Check sheet for the modelled part. Datum: model origin and axes. Units: mm. A direction names the side the tool comes from. Round coordinates to 2 decimals unless told otherwise and drop trailing zeros. Loops run counter-clockwise (first coordinate to the right, second up) from the corner with the lowest first, then second, coordinate; pieces in that order, holes last. Notation, with made-up numbers: M 35.25,14 L 93.25,14 A27 cw 93.25,53 Z; hole C -2,51.25 d6. An arc over 180 degrees is marked long. Write item = value, one per line. Start each with the question number.
(1) Cross-section at A-A on x = 17.5. Record the boundary of the cut face in (y, z), plus the area to 3 significant figures.
(2) Mould release check, pull along Y, two halves, no side actions. Record for faces 1 (the face through (-33.65, -293.89, 14.79)), 2 (the face through (16, -148, 30)), 3 (the face through (35.88, -159.72, 14.79)): pulls with the +Y half, pulls with the -Y half, needs draft (parallel to the pull), parting line crosses it, or undercut.
(3) Cross-section at C-C on x = 0. Record the boundary of the cut face in (y, z), plus the area to 3 significant figures.
(4) Set-up check for faces 4 (the face through (18, -162, 0)), 5 (the face through (13.163, -144.473, 14.79)): record each of +Z, -Z, +X, -X, +Y, -Y from which the full face is reachable in a straight line by a thin tool's end or side.
(5) Cross-section at B-B on z = 21.25. Record the boundary of the cut face in (x, y), plus the area to 3 significant figures.
(6) Cross-section at D-D on y = 0. Record the boundary of the cut face in (x, z).
(7) Scan lines: L1, parallel to X at y = -142, z = 20; L2, parallel to X at y = -294, z = 22.75; L3, parallel to Y at x = -25.5, z = 18.25. Record each from-to range of solid material in increasing order. Write a range as from..to.
(8) Go/stop test with flat-tipped pins: P1, Ø8, axis at x = 0.5, z = 26, coming from the -Y side; P2, Ø4, axis at y = -75.5, z = 7, coming from the +X side; P3, Ø5, axis at y = -108, z = 13.5, coming from the +X side. Record where each tip stops, or that it passes through.
Autodesk Inventor part; units mm, degrees
ref_plane "YZ Plane" through (0, 0, 0) normal (1, 0, 0) x (0, 1, 0)
ref_plane "XZ Plane" through (0, 0, 0) normal (0, 1, 0) x (-1, 0, 0)
ref_plane "XY Plane" through (0, 0, 0) normal (0, 0, 1) x (1, 0, 0)
sketch "Sketch1" plane through (0, 0, 0) normal (0, 0, 1) x (1, 0, 0)
  arc A0 (5.5018, -3.1706) -> (4.1426, 4.8126) centre (0, 0) ccw
  line L0 (-0.2789, 17.1872) -> (4.1426, 4.8126)
  arc A1 (-0.2789, 17.1872) -> (-5.4243, 16.3111) centre (-2.7743, 16.2955) ccw
  line L1 (-5.5018, 3.1706) -> (-5.4243, 16.3111)
  arc A2 (-5.5018, 3.1706) -> (-4.1426, -4.8126) centre (0, 0) ccw
  line L2 (-4.1426, -4.8126) -> (0.2789, -17.1872)
  arc A3 (0.2789, -17.1872) -> (5.4243, -16.3111) centre (2.7743, -16.2955) ccw
  line L3 (5.4243, -16.3111) -> (5.5018, -3.1706)
  circle A4 centre (1.7673, -10.3806) radius 0.5
  circle A5 centre (1.2638, -7.4232) radius 0.5
  circle A6 centre (0, 0) radius 4.375
  circle A7 centre (-2.2708, 13.3381) radius 0.5
  circle A8 centre (-1.7673, 10.3806) radius 0.5
  circle A9 centre (-1.2638, 7.4232) radius 0.5
  circle A10 centre (-2.7743, 16.2955) radius 0.5
  circle A11 centre (2.2708, -13.3381) radius 0.5
  circle A12 centre (2.7743, -16.2955) radius 0.5
  line L4 (0, 0) -> (2.7743, -16.2955)
  line L5 (0, 0) -> (47.7501, -296.1755)
  line L6 (0, 0) -> (23.8751, -148.0877)
  line L7 (-9.8725, -1.5917) -> (37.8776, -297.7672)
  line L8 (37.8776, -297.7672) -> (57.6226, -294.5838)
  line L9 (57.6226, -294.5838) -> (9.8725, 1.5917)
  line L10 (9.8725, 1.5917) -> (-9.8725, -1.5917)
  line L11 (-9.8725, -1.5917) -> (57.6226, -294.5838) construction
  line L12 (37.8776, -297.7672) -> (9.8725, 1.5917) construction
  circle A13 centre (0, 0) radius 25
  point P0 (13.5195, -21.0291)
  point P1 (-6.2255, -24.2124)
  dimension "d0" = 300
  dimension "d1" = 150
  dimension "d2" = 20
  dimension "d3" = 50
extrude "Extrusion1" add sketch "Sketch1" along normal blind 30 contours L3 A3 L5 A12 L4 A11 A4 A5 A6 L10 A0 | A0 L10 L9 A13 L5 A3 L3 | L10 A6 A2 L1 A1 L0 A0 | A0 L0 A1 L1 A2 L10 L7 A13 L9 | L10 A6 | A6 L4 L10 | L5 A13 L7 L10 A2 L2 A3 | A3 L2 A2 L10 A6 L5 A5 A4 A11 A12 | L9 L8 L5 A13 | L10 L5 A6 | L4 A6 L5 | L5 A12 | A12 L5 | L5 L8 L7 A13 | L4 A5 L5 A6 | L5 A11 L4 A12 | L4 A5 L5 | A5 L4 | L5 A5 | L5 A11 L4 | A11 L5 | L4 A4 L5 A5 | L4 A11 | L5 A4 L4 A11 | L4 A4 L5 | A4 L4 | L5 A4 | A7 | A8 | A9 | A10
sketch "Sketch2" plane through (37.8776, -297.7672, 0) normal (-0.9872517, -0.159167, 0) x (0, 0, 1)
  line L0 (30, 277.0871) -> (30, 0)
  line L1 (30, 0) -> (0, 0)
  line L2 (0, 0) -> (0, 30)
  line L3 (0, 30) -> (30, 30)
  line L4 (30, 30) -> (30, 0)
  point P0 (0, 300)
  point P1 (30, 30)
  dimension "d6" = 30
  dimension "d7" = 30
extrude "Extrusion2" add sketch "Sketch2" along normal blind 70
properties part number "arm" material "PET Plastic"
Result:
q1.outline = M -301.05,0 L -270.67,0 L -270.67,30 L -301.05,30 Z; M -171.37,0 L -45.72,0 L -45.72,30 L -171.37,30 Z; M -17.85,0 L 17.85,0 L 17.85,30 L -17.85,30 Z
q1.area = 5,750 mm^2
q2.face_1 = pulls with the -Y half
q2.face_2 = needs draft
q2.face_3 = undercut
q3.outline = M -303.87,0 L -273.49,0 L -273.49,30 L -303.87,30 Z; M -62.83,0 L 25,0 L 25,30 L -62.83,30 Z
q3.area = 3,550 mm^2
q4.face_4 = -Z, +X, -X, +Y, -Y
q4.face_5 = +Z, -Z, -X
q5.outline = M -36.01,-279.29 L -31.23,-308.91 L 37.88,-297.77 L 57.62,-294.58 L 13.52,-21.03 A25 ccw long -6.23,-24.21 L 33.1,-268.15 Z
q5.area = 9,580 mm^2
q6.outline = M -25,0 L 25,0 L 25,30 L -25,30 Z
q7.L1 = 12.76..33.02
q7.L2 = -33.63..57.53
q7.L3 = -307.99..-277.6
q8.P1 = -304.44
q8.P2 = 22.62
q8.P3 = 27.94
